Geometry check sheet. Reference: the model listing, model coordinates, mm. Coordinates: 2 decimals unless noted, no trailing zeros. Loops run counter-clockwise (first coordinate to the right, second up) from the corner with the lowest first, then second, coordinate; pieces in that order, holes last. Notation, with made-up numbers: (39.25, 2) - (53.25, 2) arc R32 ccw to (53.25, 41) - close; hole circle Ø3 at (45, 45.25). An arc over 180 degrees is marked (long way). One line per item, written item: value.
from build123d import *

# Parameters (mm, degrees)
F0_W     = 254
F0_H     = 25.4
F1_DEPTH = 6.35
F2_SIZE2 = 12.69999
F2_SIZE  = 6.34999


# Not quite as in the source:
# - a fillet or chamfer is up to 0.001 mm smaller than in the source, because OpenCascade refuses the exact size


with BuildPart() as f1:
    # F0 (on Front) → F1 (new body)
    with BuildSketch(Plane.XZ):
        with Locations((127, 12.7)):
            Rectangle(F0_W, F0_H)
        Polygon((-54.1485526787, 79.0131909403), (0, 25.4), (254, 25.4), (308.1485526787, 79.0131909403), align=None)
    extrude(amount=F1_DEPTH)

    # F2 (size 6.35 and 12.7 in the source; OpenCascade refuses exactly that, so slightly less here)
    f2_edges = [f1.edges().sort_by_distance(p)[0] for p in [
        (127, -6.35, 79.013191),
    ]]
    f2_side = f1.faces().sort_by_distance((127, -3.175, 79.013191))[0]
    chamfer(f2_edges, length=F2_SIZE, length2=F2_SIZE2, reference=f2_side)


solid = f1.part
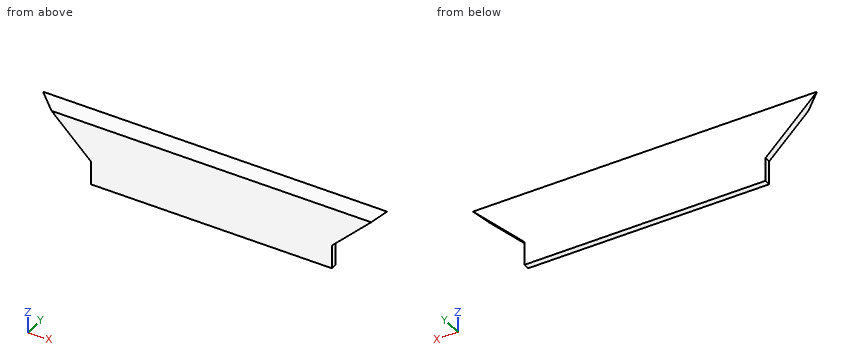
(1) Material ranges on probe 1 along X at (y, z) = (-3, 4); probe 2 along Z at (x, y) = (268, -0.75); probe 3 along X at (y, z) = (-2.75, 71), recorded low to high. Write a range as from..to.
Reply:
probe 1: 0..254
probe 2: 39.26..77.51
probe 3: -46.06..300.06
(2) Cross-section at B-B on y = -4. Record the cut outline in (x, z).
Reply:
outline: (-46.07, 71.01) - (0, 25.4) - (0, 0) - (254, 0) - (254, 25.4) - (300.07, 71.01) - close
(3) Go/stop test with flat-tipped pins: pin 1 Ø10 at (x, z) = (251, 55.5) entering from +Y; pin 2 Ø1.9 at (y, z) = (-4, 6.5) entering from -X; pin 3 Ø1 at (y, z) = (-4.5, 64.5) entering from +X. Record where each tip stops, or that it passes through.
Reply:
pin 1: y = 0
pin 2: x = 0
pin 3: x = 294
(4) Cross-section at C-C on z = 33.5. Record the cut outline in (x, y), and give its area (3 significant figures).
Reply:
outline: (-8.18, -6.35) - (262.18, -6.35) - (262.18, 0) - (-8.18, 0) - close
area: 1,720 mm2
